Build history of the part. All positions in model axes, mm. Give positions to 0.01 mm unless a question says otherwise; leave off trailing zeros. Order: outer loops, then holes, each group sorted by start corner. A loop starts at its lowest first (then second) coordinate and runs counter-clockwise, first axis right, second up. Notation, with made-up numbers: M -17.75,-14.75 L 32.25,-14.75 A7 cw 32.25,-2.75 Z; hole C 79,63.25 d5. An arc over 180 degrees is marked long. Use CSV: the item, a comma, the result in double quotes. Start each with the question number.
Item 1: Band-saw the part on C-C on z = 38. Write the cut outline in (x, y).
Item 2: Band-saw the part on B-B on y = 2.3. Give the number of separate pieces and of enclosed holes in the cut face, plus the area to 3 significant figures.
Item 3: Wall check: line 1 along X through (y, z) = (0.75, -8.25); line 2 along X through (y, z) = (2, -7); line 3 along Z through (x, y) = (67, 0.15). Give the ranges that are in metal, low to high.
Item 4: Band-saw the part on D-D on x = 23.5. Write the cut outline in (y, z), plus the area to 3 significant figures.
Item 5: Band-saw the part on A-A on x = 62.5. Write the cut outline in (y, z), plus the area to 3 significant figures.
Item 6: Pin check, flat tip, straight feed: P1, Ø3.5, axis at x = 62.5, z = 0, coming from the -Y side. Stop position of the tip, or through.
from build123d import *

# Parameters (mm, degrees)
SKETCH1_R           = 76
SKETCH1_R_2         = 1.5
SKETCH1_R_3         = 2
SKETCH1_R_4         = 3
BOSS_EXTRUDE1_DEPTH = 3


with BuildPart() as part:
    # Sketch1 → Boss-Extrude1 (new body)
    with BuildSketch(Plane(origin=(0, 0, 0), x_dir=(1, 0, 0), z_dir=(0, 1, 0))):
        with Locations(Location((0, 0, 0), (0, 0, 270))):
            Circle(SKETCH1_R)
        with Locations(Location((-65.979085433, -8.25, 0), (0, 0, 270))):
            Circle(SKETCH1_R_2, mode=Mode.SUBTRACT)
        with Locations(Location((-62.5, 0, 0), (0, 0, 270))):
            Circle(SKETCH1_R_3, mode=Mode.SUBTRACT)
        with Locations(Location((-65.979085433, 8.25, 0), (0, 0, 270))):
            Circle(SKETCH1_R_2, mode=Mode.SUBTRACT)
        with Locations(Location((65.979085433, 8.25, 0), (0, 0, 270))):
            Circle(SKETCH1_R_2, mode=Mode.SUBTRACT)
        with Locations(Location((65.979085433, -8.25, 0), (0, 0, 270))):
            Circle(SKETCH1_R_2, mode=Mode.SUBTRACT)
        with Locations(Location((0, 62.5, 0), (0, 0, 270))):
            Circle(SKETCH1_R_3, mode=Mode.SUBTRACT)
        with Locations(Location((62.5, 0, 0), (0, 0, 270))):
            Circle(SKETCH1_R_3, mode=Mode.SUBTRACT)
        with Locations(Location((0, -62.5, 0), (0, 0, 270))):
            Circle(SKETCH1_R_3, mode=Mode.SUBTRACT)
        with Locations(Location((17.5, 0, 0), (0, 0, 270))):
            Circle(SKETCH1_R_4, mode=Mode.SUBTRACT)
        with Locations(Location((-17.5, 0, 0), (0, 0, 270))):
            Circle(SKETCH1_R_4, mode=Mode.SUBTRACT)
    extrude(amount=BOSS_EXTRUDE1_DEPTH)


solid = part.part
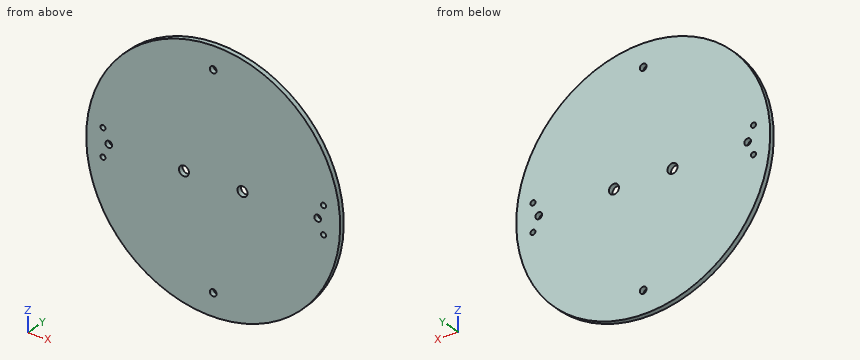
Model answer:
1,outline,"M -65.82,0 L 65.82,0 L 65.82,3 L -65.82,3 Z"
2,separate pieces,"1"
2,enclosed holes,"10"
2,area,"18,000 mm^2"
3,line 1,"x = -75.55 to -67.48, -64.48 to 64.48, 67.48 to 75.55"
3,line 2,"x = -75.68 to -66.81, -65.15 to 65.15, 66.81 to 75.68"
3,line 3,"z = -35.87 to -9.35, -7.15 to 7.15, 9.35 to 35.87"
4,outline,"M 0,-72.28 L 3,-72.28 L 3,72.28 L 0,72.28 Z"
4,area,"434 mm^2"
5,outline,"M 0,-43.24 L 3,-43.24 L 3,-2 L 0,-2 Z; M 0,2 L 3,2 L 3,43.24 L 0,43.24 Z"
5,area,"247 mm^2"
6,P1,"passes through"
